Work out the finished part from the listing and answer in its coordinate system (mm). A direction names the side the tool comes from. Coordinates: 2 decimals unless noted, no trailing zeros. Order: outer loops, then holes, each group sorted by start corner. A loop starts at its lowest first (then second) coordinate and runs counter-clockwise, first axis right, second up. Notation, with made-up numbers: (12, -19) -> (71, -19) arc R11 cw to (71, 0) -> close; hole circle Ø7 at (82, 39). An arc over 180 degrees is marked (long way). Answer as CSV lines item,"result". Start each with the question number.
Item 1: Section A-A (y = 3) is taken. Write down the section's boundary in (x, z).
Item 2: For a pull along X with two mould halves and no side action, classify faces 1 (the face through (9, -12, 0)), 2 (the face through (-8.3, -11.55, 1.29)) as pulls with the +X half, pulls with the -X half, needs draft (parallel to the pull), parting line crosses it, or undercut.
Item 3: Straight lines are drawn through the part: L1, parallel to X at y = -10, z = 1.3; L2, parallel to Y at x = -5.5, z = 1.25; L3, parallel to X at y = -26, z = 1.9. For each, find the intervals that lie inside material, in ascending order.
Item 4: Section B-B (x = 19.5) is taken. Write down the section's boundary in (y, z).
Item 5: Each of these flat-tipped pins is pushed along its axis until it touches: pin 1 Ø1.5 at (y, z) = (16.5, 1) entering from -X; pin 2 Ø1 at (x, z) = (20.5, 2) entering from -Y; pin 3 Ø1.5 at (x, z) = (-21, 1) entering from +Y. Where does it stop, or does it pass through?
Item 6: Section D-D (x = 38) is taken. Write down the section's boundary in (y, z), then the cut area to 3 significant figures.
Item 7: Section C-C (y = 22) is taken. Write down the section's boundary in (x, z), then the cut area to 3 significant figures.
Item 8: Which of the six approach directions +Z, -Z, +X, -X, +Y, -Y give full straight-line access (tool end or side, diameter ignored) to faces 3 (the face through (9, -12, 2.54)), 4 (the face through (-38.4, 2.9, 1.3))?
```python
from build123d import *

# Parameters (mm, degrees)
BOSS_EXTRUDE1_DEPTH = 2.54
CIRPATTERN1_COUNT   = 10
CUT_EXTRUDE1_REACH  = 72.152


with BuildPart() as part:
    # Sketch1 → Boss-Extrude1 (new body)
    with BuildSketch(Plane.XY):
        with BuildLine():
            Line((0, 0), (11.197309056, 15.411773743))
            ThreePointArc((11.197309056, 15.411773743), (14.528469134, 35.931399889), (0, 50.8))
            ThreePointArc((0, 50.8), (8.000279424, 39.356176552), (8.334788134, 25.39717695))
            ThreePointArc((8.334788134, 25.39717695), (5.238209343, 20.817448624), (0, 19.05))
            Line((0, 19.05), (0, 0))
        make_face()
    extrude(amount=BOSS_EXTRUDE1_DEPTH)


with BuildPart() as cirpattern1_1:
    # CirPattern1: pattern copy
    add(part.part.rotate(Axis((0, 0, 0), (0, 0, 1)), 1 * 360 / CIRPATTERN1_COUNT))


with BuildPart() as cirpattern1_2:
    # CirPattern1: pattern copy
    add(part.part.rotate(Axis((0, 0, 0), (0, 0, 1)), 2 * 360 / CIRPATTERN1_COUNT))


with BuildPart() as cirpattern1_3:
    # CirPattern1: pattern copy
    add(part.part.rotate(Axis((0, 0, 0), (0, 0, 1)), 3 * 360 / CIRPATTERN1_COUNT))


with BuildPart() as cirpattern1_4:
    # CirPattern1: pattern copy
    add(part.part.rotate(Axis((0, 0, 0), (0, 0, 1)), 4 * 360 / CIRPATTERN1_COUNT))


with BuildPart() as cirpattern1_5:
    # CirPattern1: pattern copy
    add(part.part.rotate(Axis((0, 0, 0), (0, 0, 1)), 5 * 360 / CIRPATTERN1_COUNT))


with BuildPart() as cirpattern1_6:
    # CirPattern1: pattern copy
    add(part.part.rotate(Axis((0, 0, 0), (0, 0, 1)), 6 * 360 / CIRPATTERN1_COUNT))


with BuildPart() as cirpattern1_7:
    # CirPattern1: pattern copy
    add(part.part.rotate(Axis((0, 0, 0), (0, 0, 1)), 7 * 360 / CIRPATTERN1_COUNT))


with BuildPart() as cirpattern1_8:
    # CirPattern1: pattern copy
    add(part.part.rotate(Axis((0, 0, 0), (0, 0, 1)), 8 * 360 / CIRPATTERN1_COUNT))


with BuildPart() as cirpattern1_9:
    # CirPattern1: pattern copy
    add(part.part.rotate(Axis((0, 0, 0), (0, 0, 1)), 9 * 360 / CIRPATTERN1_COUNT))


with BuildPart() as cirpattern1_8_1:
    add(cirpattern1_8.part)

    # Combine1: union CirPattern1_3, CirPattern1_7, CirPattern1_2, CirPattern1_6, part, CirPattern1_1, CirPattern1_5, CirPattern1_9, CirPattern1_4
    add(cirpattern1_3.part)
    add(cirpattern1_7.part)
    add(cirpattern1_2.part)
    add(cirpattern1_6.part)
    add(part.part)
    add(cirpattern1_1.part)
    add(cirpattern1_5.part)
    add(cirpattern1_9.part)
    add(cirpattern1_4.part)

    # Sketch2 → Cut-Extrude1 (cut, up to next)
    with BuildSketch(Plane.XY.offset(2.54), mode=Mode.PRIVATE) as cut_extrude1_sk1:
        with BuildLine():
            ThreePointArc((12.892749535, 9.36713084), (13.527827888, 4.395457728), (15.936314842, 0))
            ThreePointArc((15.936314842, 0), (13.527827888, -4.395457728), (12.892749535, -9.36713084))
            ThreePointArc((12.892749535, -9.36713084), (8.360657429, -11.507457728), (4.924592114, -15.156336076))
            ThreePointArc((4.924592114, -15.156336076), (0, -14.224), (-4.924592114, -15.156336076))
            ThreePointArc((-4.924592114, -15.156336076), (-8.360657429, -11.507457728), (-12.892749535, -9.36713084))
            ThreePointArc((-12.892749535, -9.36713084), (-13.527827888, -4.395457728), (-15.936314842, 0))
            ThreePointArc((-15.936314842, 0), (-13.527827888, 4.395457728), (-12.892749535, 9.36713084))
            ThreePointArc((-12.892749535, 9.36713084), (-8.360657429, 11.507457728), (-4.924592114, 15.156336076))
            ThreePointArc((-4.924592114, 15.156336076), (0, 14.224), (4.924592114, 15.156336076))
            ThreePointArc((4.924592114, 15.156336076), (8.360657429, 11.507457728), (12.892749535, 9.36713084))
        make_face()
    cut_extrude1_tool1 = extrude(cut_extrude1_sk1.sketch, amount=-CUT_EXTRUDE1_REACH, mode=Mode.PRIVATE) & cirpattern1_8_1.part
    add(cut_extrude1_tool1.solids().sort_by_distance((0, 0, 2.54))[0], mode=Mode.SUBTRACT)


solid = cirpattern1_8_1.part
```
Checked values:
1,outline,"(-38.25, 0) -> (-14.07, 0) -> (-14.07, 2.54) -> (-38.25, 2.54) -> close; (14.07, 0) -> (19.72, 0) -> (19.72, 2.54) -> (14.07, 2.54) -> close; (37.49, 0) -> (44.27, 0) -> (44.27, 2.54) -> (37.49, 2.54) -> close"
2,face 1,"needs draft"
2,face 2,"undercut"
3,L1,"x = -47.51 to -45.29, -25.63 to -11.03, 11.03 to 17.82"
3,L2,"y = -48.05 to -44.68, -21.02 to -14.33, 14.33 to 34"
3,L3,"x = -33.99 to -29.21, -15.41 to -8.49, 1.07 to 8.4"
4,outline,"(-41.84, 0) -> (-38.31, 0) -> (-38.31, 2.54) -> (-41.84, 2.54) -> close; (-22.46, 0) -> (-13.85, 0) -> (-13.85, 2.54) -> (-22.46, 2.54) -> close; (-6.29, 0) -> (3.27, 0) -> (3.27, 2.54) -> (-6.29, 2.54) -> close; (6.39, 0) -> (14.38, 0) -> (14.38, 2.54) -> (6.39, 2.54) -> close"
5,pin 1,"stops at x = -48.27"
5,pin 2,"stops at y = -42.03"
5,pin 3,"stops at y = 42.08"
6,outline,"(-23.44, 0) -> (-19.57, 0) -> (-19.57, 2.54) -> (-23.44, 2.54) -> close; (-3.17, 0) -> (3.3, 0) -> (3.3, 2.54) -> (-3.17, 2.54) -> close"
6,area,"26.3 mm^2"
7,outline,"(-41.1, 0) -> (-18.62, 0) -> (-18.62, 2.54) -> (-41.1, 2.54) -> close; (-7.64, 0) -> (-0.19, 0) -> (-0.19, 2.54) -> (-7.64, 2.54) -> close; (6.5, 0) -> (14.52, 0) -> (14.52, 2.54) -> (6.5, 2.54) -> close; (27.26, 0) -> (33.31, 0) -> (33.31, 2.54) -> (27.26, 2.54) -> close"
7,area,"112 mm^2"
8,face 3,"+Z, +X, -X, +Y, -Y"
8,face 4,"+Z, -Z"
